Design review of the part built by this model. Coordinates are the model's own, in mm. A direction names the side the tool comes from. Round coordinates to 2 decimals unless told otherwise and drop trailing zeros. Loops run counter-clockwise (first coordinate to the right, second up) from the corner with the lowest first, then second, coordinate; pieces in that order, holes last. Notation, with made-up numbers: M 86.25,82 L 120.25,82 A23 cw 120.25,96 Z; hole C 7,70.25 d7. An arc over 180 degrees is marked long. Use a Markdown table: item, result.
from build123d import *

# Parameters (mm, degrees)
F1_DEPTH = 4.7752
F2_R     = 3.96875
F3_DEPTH = 4.7762
F4_R     = 4.7625
F5_DEPTH = 4.7762
F6_SIZE  = 0.381
F7_SIZE  = 0.381


with BuildPart() as f1:
    # F0 (on Top) → F1 (new body)
    with BuildSketch(Plane.XY):
        with BuildLine():
            ThreePointArc((20.216247, -1.591479), (21.680928, -1.971354), (22.803448, -2.986018))
            ThreePointArc((22.803448, -2.986018), (37.312981, 1.381884), (22.897449, 6.050669))
            ThreePointArc((22.897449, 6.050669), (21.783346, 5.074773), (20.347779, 4.710432))
            Line((20.347779, 4.710432), (-35.892979, 3.971447))
            ThreePointArc((-35.892979, 3.971447), (-37.359656, 4.308902), (-38.506159, 5.283865))
            ThreePointArc((-38.506159, 5.283865), (-49.999089, 1.559265), (-38.506178, -2.165395))
            ThreePointArc((-38.506178, -2.165395), (-37.359647, -1.190426), (-35.892939, -0.852992))
            Line((-35.892939, -0.852992), (20.216247, -1.591479))
        make_face()
    extrude(amount=F1_DEPTH)

    # F2 (on face) → F3 (cut, through all)
    with BuildSketch(Plane.XY.offset(4.7752)):
        with Locations((-43.649089, 1.559248)):
            Circle(F2_R)
    extrude(amount=-F3_DEPTH, mode=Mode.SUBTRACT)

    # F4 (on face) → F5 (cut, through all)
    with BuildSketch(Plane.XY.offset(4.7752)):
        with Locations((29.375911, 1.464447)):
            Circle(F4_R)
    extrude(amount=-F5_DEPTH, mode=Mode.SUBTRACT)

    # F6
    f6_edges = [f1.edges().sort_by_distance(p)[0] for p in [
        (37.312981, 1.381884, 4.7752),
        (21.783346, 5.074773, 4.7752),
        (-7.7726, 4.34094, 4.7752),
        (21.680928, -1.971354, 4.7752),
        (-7.838346, -1.222235, 4.7752),
        (-37.359656, 4.308902, 4.7752),
        (-49.999089, 1.559265, 4.7752),
        (-37.359647, -1.190426, 4.7752),
    ]]
    chamfer(f6_edges, length=F6_SIZE)

    # F7
    f7_edges = [f1.edges().sort_by_distance(p)[0] for p in [
        (-49.999089, 1.559265, 0),
        (-37.359647, -1.190426, 0),
        (-37.359656, 4.308902, 0),
        (-7.838346, -1.222235, 0),
        (-7.7726, 4.34094, 0),
        (21.680928, -1.971354, 0),
        (37.312981, 1.381884, 0),
        (21.783346, 5.074773, 0),
    ]]
    chamfer(f7_edges, length=F7_SIZE)


solid = f1.part
1. Insertion check: pin 1 (1.5 mm diameter, centred on y = -2.5, z = 3.5, fed in from +X); pin 2 (2 mm diameter, centred on y = 4.5, z = 3, fed in from +X); pin 3 (1.5 mm diameter, centred on x = 7, y = -2.5, fed in from -Z); pin 4 (1 mm diameter, centred on x = 3, z = 1, fed in from -Y). Each pin has a flat end and moves straight along its axis. Give the tip position at first contact, or say it passes through.
Check values:
| item | result |
|---|---|
| pin 1 | stops at x = 36.63 |
| pin 2 | stops at x = 37.05 |
| pin 3 | passes through |
| pin 4 | stops at y = -1.37 |
2. Machinability: for faces 1 (the face through (33.92, 2.89, 2.42)), 2 (the face through (21.66, -1.96, 2.36)), 3 (the face through (21.802, 5.085, 2.36)), which of the approach directions +Z, -Z, +X, -X, +Y, -Y give a long, thin tool a straight path to every point of the face, cutting with its end or side? Answer none if there is none.
Check values:
| item | result |
|---|---|
| face 1 | +Z, -Z |
| face 2 | +Z, -Z, -Y |
| face 3 | +Z, -Z, +Y |
3. Wall thickness on line 1 along Y through (x, z) = (29, 2); line 2 along X through (y, z) = (0.5, 4.65); line 3 along X through (y, z) = (-2.75, 1.55): over which ranges is each line inside the solid? List them lowest first. Write a range as from..to.
Check values:
| item | result |
|---|---|
| line 1 | y = -6.46..-3.28, 6.21..9.39 |
| line 2 | x = -49.65..-47.47, -39.82..24.71, 34.04..37 |
| line 3 | x = -48.31..-38.99, 22.63..27.16, 31.59..36.1 |
4. Take a section at A-A on z = 2.4. Count the separate pieces of the cut face and the enclosed holes in it, and give its area (3 significant figures).
Check values:
| item | result |
|---|---|
| separate pieces | 1 |
| enclosed holes | 2 |
| area | 535 mm² |
5. Take a section at B-B on x = -13.5. Give the boundary of the cut face in (y, z), and give its area (3 significant figures).
Check values:
| item | result |
|---|---|
| outline | M -1.15,0.38 L -0.77,0 L 3.88,0 L 4.27,0.38 L 4.27,4.39 L 3.88,4.78 L -0.77,4.78 L -1.15,4.39 Z |
| area | 25.6 mm² |
6. The part is to be moulded in two halves that separate along X. For faces 4 (the face through (-3, 1, 4.775)), 5 (the face through (-37.34, 4.3, 2.36)), say which applies: pulls with the +X half, pulls with the -X half, needs draft (parallel to the pull), parting line crosses it, or undercut.
Check values:
| item | result |
|---|---|
| face 4 | needs draft |
| face 5 | undercut |
